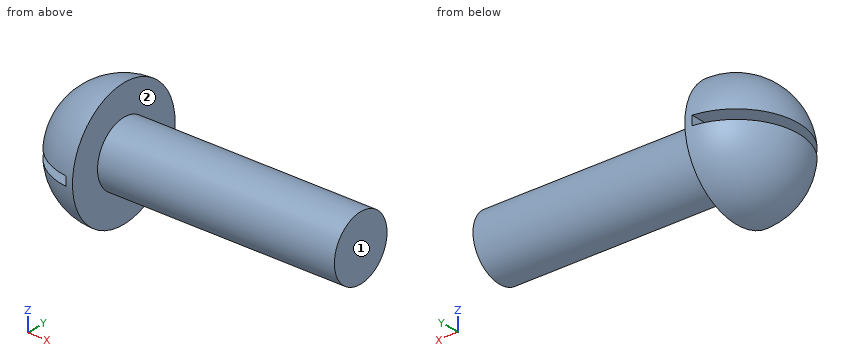
from build123d import *

# Parameters (mm, degrees)
SKETCH2_W          = 0.5
SKETCH2_H          = 8.749412665
CUT_EXTRUDE1_DEPTH = 3


with BuildPart() as part:
    # Sketch1 → Revolve3 (revolve)
    with BuildSketch(Plane.XY):
        with BuildLine():
            Line((12.7, 0), (12.7, 1.7272))
            Line((12.7, 1.7272), (0, 1.7272))
            Line((0, 1.7272), (0, 3.371476925))
            ThreePointArc((0, 3.371476925), (-2.383994197, 2.383994197), (-3.371476925, 0))
            Line((-3.371476925, 0), (12.7, 0))
        make_face()
    revolve(axis=Axis((25.331759203, 0, 0), (-1, 0, 0)))

    # Sketch2 → Cut-Extrude1 (cut)
    with BuildSketch(Plane.ZY.offset(3.371476925)):
        with Locations((0, -0.032949338)):
            Rectangle(SKETCH2_W, SKETCH2_H)
    extrude(amount=-CUT_EXTRUDE1_DEPTH, mode=Mode.SUBTRACT)


solid = part.part
For this review, take the finished solid that the model builds, in its own axes (mm). Face numbers are marked on the shaded views. A direction names the side the tool comes from. Round coordinates to 2 decimals unless told otherwise and drop trailing zeros. Write each loop counter-clockwise with the first axis right and the second up, starting at its lowest first coordinate (ties: lowest second). Pieces come first, ordered by that corner, then holes. Notation, with made-up numbers: (-36.75, 20.25) -> (6.25, 20.25) arc R26 cw to (6.25, 57.25) -> close; hole circle Ø11 at (-6.75, 30.5). An arc over 180 degrees is marked (long way). Use CSV: the item, a comma, the result in double quotes.
(1) For the marked faces 1 and 2, list the 3-axis set-ups (+Z, -Z, +X, -X, +Y, -Y) from which the entire face can be reached by the end or side of a thin tool; tool diameter is ignored.
Computed values:
face 1,"+Z, -Z, +X, +Y, -Y"
face 2,"+X"
(2) Consider section C-C, the plane x = 3.25. Give the boundary of the cut face in (y, z).
Computed values:
outline,"circle Ø3.45 at (0, 0)"
(3) Consider section B-B, the plane z = -1.5. Give the boundary of the cut face in (x, y), plus the area to 3 significant figures.
Computed values:
outline,"(0, -3.02) -> (0, -0.86) -> (12.7, -0.86) -> (12.7, 0.86) -> (0, 0.86) -> (0, 3.02) arc R3.02 ccw to start"
area,"36.1 mm²"
(4) Consider section D-D, the plane y = 1. Give the boundary of the cut face in (x, z).
Computed values:
outline,"(-3.21, -0.25) arc R3.22 ccw to (0, -3.22) -> (0, -1.41) -> (12.7, -1.41) -> (12.7, 1.41) -> (0, 1.41) -> (0, 3.22) arc R3.22 ccw to (-3.21, 0.25) -> (-0.37, 0.25) -> (-0.37, -0.25) -> close"
(5) To check wall thickness, follow L1, parallel to Y at x = 5.25, z = 0; L2, parallel to Z at x = -1, y = -2.5; L3, parallel to X at y = 1.25, z = 0. State the ranges of each line that lie inside material, in increasing order. Write a range as [from, to].
Computed values:
L1,"[-1.73, 1.73]"
L2,"[-2.03, -0.25], [0.25, 2.03]"
L3,"[-0.37, 12.7]"
(6) Clearance check with flat-ended pins moving along their axes: P1, Ø1.5, axis at x = -1.5, y = -0.5, coming from the +Z side; P2, Ø4, axis at x = 8, y = 1, coming from the -Z side; P3, Ø4, axis at x = 7.5, z = -2.5, coming from the -Y side. State where each tip first meets the part, or that it passes through.
Computed values:
P1,"z = 3.27"
P2,"z = -1.73"
P3,"y = -1.65"
(7) Consider section A-A, the plane y = 0. Give the boundary of the cut face in (x, z), plus the area to 3 significant figures.
Computed values:
outline,"(-3.36, -0.25) arc R3.37 ccw to (0, -3.37) -> (0, -1.73) -> (12.7, -1.73) -> (12.7, 1.73) -> (0, 1.73) -> (0, 3.37) arc R3.37 ccw to (-3.36, 0.25) -> (-0.37, 0.25) -> (-0.37, -0.25) -> close"
area,"60.2 mm²"
